```python
from build123d import *

# Parameters (mm, degrees)
F1_DEPTH     = 20
F2_R         = 1.6
F2_R_2       = 5.175
F3_DEPTH     = 7
F4_DEPTH     = 25
F5_R         = 3
F6_T1_DEPTH  = 28.6148731674
F7_DEPTH     = 25
F9_DEPTH     = 25
F10_T1_DEPTH = 35.1990481771


# Not quite as in the source:
# - a fillet or chamfer that OpenCascade refuses, or shapes differently, is made with other operations: its cross-section is extruded or revolved along the edge and cut away or added
# - a feature names something its author has since deleted; it is built from what else it names


with BuildPart() as f1:
    # F0 (on Front) → F1 (new body)
    with BuildSketch(Plane.XZ):
        with BuildLine():
            Line((-25, -4.125), (25, -4.125))
            Line((25, -4.125), (25, 4.125))
            Line((25, 4.125), (-5.9433734098, 4.125))
            ThreePointArc((-5.9433734098, 4.125), (-15, 9.8850100464), (-24.0566265902, 4.125))
            Line((-24.0566265902, 4.125), (-25, 4.125))
            Line((-25, 4.125), (-25, -4.125))
        make_face()
    extrude(amount=F1_DEPTH)

    # F2 (on face) → F3 (cut)
    with BuildSketch(Plane(origin=(0, 0, -4.125), x_dir=(1, 0, 0), z_dir=(0, 0, -1))):
        with Locations((-22.5875, 10)):
            Circle(F2_R)
        with Locations((-15, 10)):
            Circle(F2_R_2)
        with Locations((-15, 17.5875)):
            Circle(F2_R)
        with Locations((-15, 2.4125)):
            Circle(F2_R)
        with Locations((-7.4125, 10)):
            Circle(F2_R)
    extrude(amount=-F3_DEPTH, mode=Mode.SUBTRACT)

    # F4 (cut): a face of the model
    f4_faces = [f1.faces().sort_by_distance(p)[0] for p in [
        (-15, -10, 2.875),
    ]]
    extrude(f4_faces, amount=-F4_DEPTH, mode=Mode.SUBTRACT)

    # F5
    f5_edges = [f1.edges().sort_by_distance(p)[0] for p in [
        (25, 0, 0),
        (25, -20, 0),
        (-25, 0, 0),
        (-25, -20, 0),
    ]]
    fillet(f5_edges, radius=F5_R)

    # F6: fillet of radius 5 on 1 edges, made by hand

    # F6_s2 → F6_t1 (cut)
    with BuildSketch(Plane.XZ.offset(-4.3074365837)):
        with BuildLine():
            ThreePointArc((-24.0566265902, 4.125), (-24.7583155082, 2.7377445871), (-25, 1.2020253665))
            Line((-25, 1.2020253665), (-25, 4.125))
            Line((-25, 4.125), (-24.0566265902, 4.125))
        make_face()
    extrude(amount=F6_T1_DEPTH, mode=Mode.SUBTRACT)

    # F2 (on face) → F7 (cut)
    with BuildSketch(Plane(origin=(0, 0, -4.125), x_dir=(1, 0, 0), z_dir=(0, 0, -1))):
        with BuildLine():
            Line((25, 4.85), (25, 15.15))
            Line((25, 15.15), (11.0150124379, 15.15))
            ThreePointArc((11.0150124379, 15.15), (6.7728579207, 10), (11.0150124379, 4.85))
            Line((11.0150124379, 4.85), (25, 4.85))
        make_face()
    extrude(amount=-F7_DEPTH, mode=Mode.SUBTRACT)

    # F8 (on face) → F9 (cut)
    with BuildSketch(Plane.XZ.offset(20)):
        with BuildLine():
            Line((-21.3318682487, 7.625), (-8.6681317513, 7.625))
            ThreePointArc((-8.6681317513, 7.625), (-15, 9.8850100464), (-21.3318682487, 7.625))
        make_face()
    extrude(amount=-F9_DEPTH, mode=Mode.SUBTRACT)

    # F10: fillet of radius 5 on 2 edges, made by hand

    # F10_s2 → F10_t1 (cut)
    with BuildSketch(Plane.XZ.offset(-7.5995240885)):
        with BuildLine():
            ThreePointArc((-19.182398242, 7.625), (-21.55937639, 7.0238606347), (-23.3647964839, 5.3649899536))
            ThreePointArc((-23.3647964839, 5.3649899536), (-22.4347091347, 6.5726927603), (-21.3318682487, 7.625))
            Line((-21.3318682487, 7.625), (-19.182398242, 7.625))
        make_face()
        with BuildLine():
            ThreePointArc((-6.6352035161, 5.3649899536), (-8.44062361, 7.0238606347), (-10.817601758, 7.625))
            Line((-10.817601758, 7.625), (-8.6681317513, 7.625))
            ThreePointArc((-8.6681317513, 7.625), (-7.5652908653, 6.5726927603), (-6.6352035161, 5.3649899536))
        make_face()
    extrude(amount=F10_T1_DEPTH, mode=Mode.SUBTRACT)


solid = f1.part
```
Work out the finished part from the listing and answer in its coordinate system (mm). A direction names the side the tool comes from. Give positions to 0.01 mm unless a question says otherwise; leave off trailing zeros. Loops run counter-clockwise (first coordinate to the right, second up) from the corner with the lowest first, then second, coordinate; pieces in that order, holes last. Notation, with made-up numbers: M -19.75,87 L 39.25,87 A19 ccw 39.25,106 Z; hole C 66.25,19 d6. An arc over 180 degrees is marked long. One line per item, written item: value. Start each with the question number.
1. Find section C-C (y = -7.5). Give the vertices of the cut face in (x, z) (3 decimals).
2. Find the intervals of material crossed by probe 1 along X at (y, z) = (-10, -2.5) (1 decimal); probe 2 along Y at (x, z) = (16, -3.5); probe 3 along Y at (x, z) = (-14, 0), in increasing order.
3. Find section B-B (z = -2). State how many separate pieces and enclosed holes the cut face has, and give its area (3 significant figures).
4. Which of the six approach directions +Z, -Z, +X, -X, +Y, -Y give full straight-line access (tool end or side, diameter ignored) to faces 5 (the face through (-23.728, -9.865, 4.766)), 6 (the face through (-16.27, -16.614, -0.674))?
5. Find section A-A (x = 12.5). Give the vertices of the cut face in (y, z) (3 decimals), and give its area (3 significant figures).
6. Determine the mould class of faces 1 (the face through (24.14, -19.1, 0.06)), 2 (the face through (6.774, -10.101, -0.058)), 3 (the face through (18, -15.15, 0)), 4 (the face through (-21.53, -9.86, 7.04)) for opening direction Y: released by +Y, released by -Y, zero draft, split by the parting line, or undercut.
7. Find section D-D (x = -15). Give the vertices of the cut face in (y, z) (1 decimal).
8. This flat-tipped pin is pushed along its axis until it touches: P1, Ø1, axis at x = -14.5, y = -18, coming from the -Z side (3 decimals). Where does it stop, or does it pass through?
Reported:
1. outline: M -25,-4.125 L -19.531,-4.125 L -19.531,7.613 A5 ccw -23.365,5.365 A10 ccw -24.057,4.125 A5 ccw -25,1.202 Z; M -10.469,-4.125 L 7.407,-4.125 L 7.407,4.125 L -5.943,4.125 A10 ccw -6.635,5.365 A5 ccw -10.469,7.613 Z
2. probe 1: x = -25 to -24.2, -21 to -20.2, -9.8 to -9, -5.8 to 6.8
2. probe 2: y = -20 to -15.15, -4.85 to 0
2. probe 3: y = -20 to -18.84, -16.34 to -15.08, -4.92 to -3.66, -1.16 to 0
3. separate pieces: 1
3. enclosed holes: 5
3. area: 699 mm²
4. face 5: +Z, -X, +Y, -Y
4. face 6: -Z
5. outline: M -20,-4.125 L -15.15,-4.125 L -15.15,4.125 L -20,4.125 Z; M -4.85,-4.125 L 0,-4.125 L 0,4.125 L -4.85,4.125 Z
5. area: 80.0 mm²
6. face 1: released by -Y
6. face 2: undercut
6. face 3: undercut
6. face 4: zero draft
7. outline: M -20,-4.1 L -19.2,-4.1 L -19.2,2.9 L -16,2.9 L -16,-4.1 L -15.2,-4.1 L -15.2,7.6 L -20,7.6 Z; M -4.8,-4.1 L -4,-4.1 L -4,2.9 L -0.8,2.9 L -0.8,-4.1 L 0,-4.1 L 0,7.6 L -4.8,7.6 Z
8. P1: stops at z = 2.875
